Model file for the job. Use its own axes, mm. A direction names the side the tool comes from. Give positions to 0.01 mm unless a question says otherwise; leave off trailing zeros. Write each loop counter-clockwise with the first axis right and the second up, starting at its lowest first coordinate (ties: lowest second). Pieces come first, ordered by that corner, then holes. Notation, with made-up numbers: (61.5, 45.5) - (103.5, 45.5) arc R9 cw to (103.5, 55.5) - close; hole circle Ø5 at (-21, 37). An arc over 180 degrees is marked (long way). Use CSV: the item, a comma, the result in double quotes.
from build123d import *

# Parameters (mm, degrees)
SKETCH_W     = 55
SKETCH_H     = 48
PAD_DEPTH    = 1.5
SKETCH001_R  = 3.85
PAD001_DEPTH = 6
SKETCH002_R  = 1.375
POCKET_DEPTH = 6
PAD002_DEPTH = 10
SKETCH004_W  = 42
SKETCH004_H  = 1.5
PAD003_DEPTH = 8


with BuildPart() as part:
    # Sketch → Pad (new body)
    with BuildSketch(Plane.XY):
        with Locations((27.5, 24)):
            Rectangle(SKETCH_W, SKETCH_H)
    extrude(amount=PAD_DEPTH)

    # Sketch001 (on Face6 of Pad) → Pad001 (join)
    with BuildSketch(Plane.XY.offset(1.5)):
        with Locations((6.6, 6.6)):
            Circle(SKETCH001_R)
        with Locations((6.6, 40.6)):
            Circle(SKETCH001_R)
        with Locations((48.6, 40.6)):
            Circle(SKETCH001_R)
        with Locations((48.6, 6.6)):
            Circle(SKETCH001_R)
    extrude(amount=PAD001_DEPTH)

    # Sketch002 (on Face11 of Pad001) → Pocket (cut)
    with BuildSketch(Plane.XY.offset(7.5)):
        with Locations((6.6, 6.6)):
            Circle(SKETCH002_R)
        with Locations((6.6, 40.6)):
            Circle(SKETCH002_R)
        with Locations((48.6, 40.6)):
            Circle(SKETCH002_R)
        with Locations((48.6, 6.6)):
            Circle(SKETCH002_R)
    extrude(amount=-POCKET_DEPTH, mode=Mode.SUBTRACT)

    # Sketch003 (on Face5 of Pocket) → Pad002 (join)
    with BuildSketch(Plane.XY.offset(1.5)):
        Polygon((0, 0), (0, 48), (55, 48), (55, 0), (48.5, 0), (48.5, 1.5), (53.5, 1.5), (53.5, 46.5), (1.5, 46.5), (1.5, 1.5), (6.5, 1.5), (6.5, 0), align=None)
    extrude(amount=PAD002_DEPTH)

    # Sketch004 (on Face8 of Pad002) → Pad003 (join)
    with BuildSketch(Plane.XY.offset(1.5)):
        with Locations((27.5, 0.75)):
            Rectangle(SKETCH004_W, SKETCH004_H)
    extrude(amount=PAD003_DEPTH)


solid = part.part
(1) Wall check: probe 1 along Y at (x, z) = (48.6, 4.9) (3 decimals); probe 2 along X at (y, z) = (3.5, 8); probe 3 along Y at (x, z) = (20, 6.75). Give the ranges that are in metal, low to high. Write a range as [from, to].
Checked values:
probe 1,"y = [0, 1.5], [2.75, 5.225], [7.975, 10.45], [36.75, 39.225], [41.975, 44.45], [46.5, 48]"
probe 2,"x = [0, 1.5], [53.5, 55]"
probe 3,"y = [0, 1.5], [46.5, 48]"
(2) Saw through at A-A, the plane z = 6.5. Count the separate pieces of the cut face and the enclosed holes in it, then the cut area to 3 significant figures.
Checked values:
separate pieces,"5"
enclosed holes,"5"
area,"463 mm^2"
(3) Pull direction X, two halves, no side cores. Call faces 1 (the face through (55, 24, 6)), 2 (the face through (27, 24, 0)), 3 (the face through (8.3, 6.7, 7.5)): released by +X, released by -X, zero draft, split by the parting line, or undercut.
Checked values:
face 1,"released by +X"
face 2,"zero draft"
face 3,"undercut"
(4) Saw through at B-B, the plane x = 41. List the corners of the cut face in (y, z), then the cut area to 3 significant figures.
Checked values:
outline,"(0, 0) - (48, 0) - (48, 11.5) - (46.5, 11.5) - (46.5, 1.5) - (1.5, 1.5) - (1.5, 9.5) - (0, 9.5) - close"
area,"99.0 mm^2"
(5) Saw through at C-C, the plane y = 6.6. List the corners of the cut face in (x, z) (3 decimals), then the cut area to 3 significant figures.
Checked values:
outline,"(0, 0) - (55, 0) - (55, 11.5) - (53.5, 11.5) - (53.5, 1.5) - (52.45, 1.5) - (52.45, 7.5) - (49.975, 7.5) - (49.975, 1.5) - (47.225, 1.5) - (47.225, 7.5) - (44.75, 7.5) - (44.75, 1.5) - (10.45, 1.5) - (10.45, 7.5) - (7.975, 7.5) - (7.975, 1.5) - (5.225, 1.5) - (5.225, 7.5) - (2.75, 7.5) - (2.75, 1.5) - (1.5, 1.5) - (1.5, 11.5) - (0, 11.5) - close"
area,"172 mm^2"
(6) Flat gauge pins, fed straight in: P1, Ø2.5, axis at x = 50.5, y = 7, coming from the +Z side; P2, Ø0.8, axis at x = 29.5, y = 1, coming from the +Z side; P3, Ø2, axis at x = 33.5, y = 16.5, coming from the +Z side. Where does each tip first touch, or does it go through?
Checked values:
P1,"stops at z = 7.5"
P2,"stops at z = 9.5"
P3,"stops at z = 1.5"
(7) 3-axis set-ups, long thin cutter, end or side, ignore diameter. For faces 4 (the face through (47.587, 41.529, 4.542)), 5 (the face through (27, 0, 4)): which of +Z, -Z, +X, -X, +Y, -Y reach the whole face in a straight line?
Checked values:
face 4,"+Z"
face 5,"+Z, -Z, +X, -X, -Y"
(8) Saw through at D-D, the plane y = 29. List the corners of the cut face in (x, z).
Checked values:
outline,"(0, 0) - (55, 0) - (55, 11.5) - (53.5, 11.5) - (53.5, 1.5) - (1.5, 1.5) - (1.5, 11.5) - (0, 11.5) - close"
